from build123d import *

# Parameters (mm, degrees)
CROQUIS1_R              = 10
SALIENTE_EXTRUIR1_DEPTH = 10
CORTAR_EXTRUIR1_DEPTH   = 5
CROQUIS3_R              = 0.6
CORTAR_EXTRUIR2_DEPTH   = 10
CROQUIS4_R              = 3
CORTAR_EXTRUIR3_DEPTH   = 5
CROQUIS5_R              = 3
CORTAR_EXTRUIR4_DEPTH   = 4


with BuildPart() as part:
    # Croquis1 → Saliente-Extruir1 (new body)
    with BuildSketch(Plane(origin=(0, 0, 0), x_dir=(1, 0, 0), z_dir=(0, 1, 0))):
        Circle(CROQUIS1_R)
    extrude(amount=SALIENTE_EXTRUIR1_DEPTH)

    # Croquis2 → Cortar-Extruir1 (cut)
    with BuildSketch(Plane.XZ):
        Polygon((5, 0), (2.5, 4.330127019), (-2.5, 4.330127019), (-5, 0), (-2.5, -4.330127019), (2.5, -4.330127019), align=None)
    extrude(amount=-CORTAR_EXTRUIR1_DEPTH, mode=Mode.SUBTRACT)

    # Croquis3 → Cortar-Extruir2 (cut)
    with BuildSketch(Plane.XZ):
        with Locations((-6.247955751, 4.354658302)):
            Circle(CROQUIS3_R)
        with Locations((6.247955751, -4.354658302)):
            Circle(CROQUIS3_R)
        with Locations((4.354658302, 6.247955751)):
            Circle(CROQUIS3_R)
        with Locations((-4.354658302, -6.247955751)):
            Circle(CROQUIS3_R)
    extrude(amount=-CORTAR_EXTRUIR2_DEPTH, mode=Mode.SUBTRACT)

    # Croquis4 → Cortar-Extruir3 (cut)
    with BuildSketch(Plane(origin=(0, 10, 0), x_dir=(1, 0, 0), z_dir=(0, 1, 0))):
        Circle(CROQUIS4_R)
    extrude(amount=-CORTAR_EXTRUIR3_DEPTH, mode=Mode.SUBTRACT)

    # Croquis5 → Cortar-Extruir4 (cut)
    with BuildSketch(Plane(origin=(0, 10, 0), x_dir=(1, 0, 0), z_dir=(0, 1, 0))):
        with Locations((6.247955751, 4.354658302)):
            Circle(CROQUIS5_R)
        with Locations((-4.354658302, 6.247955751)):
            Circle(CROQUIS5_R)
        with Locations((-6.247955751, -4.354658302)):
            Circle(CROQUIS5_R)
        with Locations((4.354658302, -6.247955751)):
            Circle(CROQUIS5_R)
    extrude(amount=-CORTAR_EXTRUIR4_DEPTH, mode=Mode.SUBTRACT)


solid = part.part
CAD build for the part. Positions are in the model's coordinates, mm. A direction names the side the tool comes from. Round coordinates to 2 decimals unless told otherwise and drop trailing zeros. Write each loop counter-clockwise with the first axis right and the second up, starting at its lowest first coordinate (ties: lowest second). Pieces come first, ordered by that corner, then holes. Notation, with made-up numbers: M -16.75,-39 L 0.25,-39 A17 cw 0.25,-22 Z; hole C 69,30 d7. An arc over 180 degrees is marked long. Put each result on its own line as item: value. Start each with the question number.
1) Pin check, flat tips, straight feed: pin 1 Ø1 at (x, z) = (-4.35, -6.25) entering from +Y; pin 2 Ø1.8 at (x, z) = (-4, -5) entering from +Y; pin 3 Ø3 at (x, z) = (-2, -1.5) entering from -Y; pin 4 Ø1.5 at (x, y) = (-1, 3) entering from +Z. Stop position of each tip, or through.
2) Saw through at C-C, the plane y = 6.25. Write the cut outline in (x, z), and give its area (3 significant figures).
3) 3-axis set-ups, long thin cutter, end or side, ignore diameter. For faces 4 (the flat face through (3.73, 2.46, -2.2)), 5 (the cylindrical face through (-3.731, 8.028, 2.722)), 6 (the flat face through (2.1, 10, -2.4)): which of +Z, -Z, +X, -X, +Y, -Y reach the whole face in a straight line?
4) Saw through at D-D, the plane y = 2.75. Write the cut outline in (x, z).
5) Saw through at B-B, the plane z = 2.5. Write the cut outline in (x, y).
6) Saw through at A-A, the plane x = 0. Write the cut outline in (y, z).
7) Pull direction Z, two halves, no side cores. Call faces 1 (the cylindrical face through (-3, 8, 0)), 2 (the flat face through (0, 0, -5)), 3 (the cylindrical face through (-1.302, 4.93, -9.915)): pulls with the +Z half, pulls with the -Z half, needs draft (parallel to the pull), parting line crosses it, or undercut.
8) Drill centre lines: probe 1 along X at (y, z) = (8.65, 0); probe 2 along X at (y, z) = (6.5, -2.5). Where is each one in solid material? Low to high. Write a range as [from, to].
Resolved:
1. pin 1: through
1. pin 2: y = 6
1. pin 3: y = 5
1. pin 4: z = 10
2. outline: M -9.21,3.89 A10 ccw -7.3,-6.84 A3 cw long -3.89,-9.21 A10 ccw 6.84,-7.3 A3 cw long 9.21,-3.89 A10 ccw 7.3,6.84 A3 cw long 3.89,9.21 A10 ccw -6.84,7.3 A3 cw long Z; hole C 0,0 d6
2. area: 180 mm²
3. face 4: -Y
3. face 5: +Y
3. face 6: +Z, -Z, +X, -X, +Y
4. outline: C 0,0 d20; hole C -6.25,4.35 d1.2; hole M -5,0 L -2.5,-4.33 L 2.5,-4.33 L 5,0 L 2.5,4.33 L -2.5,4.33 Z; hole C -4.35,-6.25 d1.2; hole C 4.35,6.25 d1.2; hole C 6.25,-4.35 d1.2
5. outline: M -9.68,0 L -3.56,0 L -3.56,5 L -1.66,5 L -1.66,10 L -3.89,10 L -3.89,6 L -8.61,6 L -8.61,10 L -9.68,10 Z; M 1.66,5 L 3.56,5 L 3.56,0 L 9.68,0 L 9.68,10 L 1.66,10 Z
6. outline: M 0,-10 L 10,-10 L 10,-3 L 5,-3 L 5,-4.33 L 0,-4.33 Z; M 0,4.33 L 5,4.33 L 5,3 L 10,3 L 10,10 L 0,10 Z
7. face 1: undercut
7. face 2: needs draft
7. face 3: parting line crosses it
8. probe 1: [-10, -3], [3, 10]
8. probe 2: [-9.68, -1.66], [1.66, 3.89], [8.61, 9.68]
